Work out the finished part from the listing and answer in its coordinate system (mm). Face numbers are marked on the shaded views. A direction names the side the tool comes from. Give positions to 0.01 mm unless a question says otherwise; leave off trailing zeros. Write each loop counter-clockwise with the first axis right and the second up, starting at its lowest first coordinate (ties: lowest second). Pieces come first, ordered by that corner, then holes.
1) Given pin 1 Ø3 at (y, z) = (6, -1) entering from +X; pin 2 Ø1 at (y, z) = (3.5, 0.5) entering from -X; pin 3 Ø1.5 at (x, z) = (-0.5, -1) entering from +Y, each flat-ended and moving along its own axis, determine where each tip first touches the part or whether it passes through.
2) Determine the mould class of the marked faces 3, 4 and 5 for opening direction Z: pulls with the +Z half, pulls with the -Z half, needs draft (parallel to the pull), parting line crosses it, or undercut.
3) A tool of negligible diameter and unlimited length cuts with its end or side. For the marked faces 1 and 2, from which of +Z, -Z, +X, -X, +Y, -Y can it reach the whole face along a straight path? Write none if from no direction.
4) Find section A-A (y = 14.5). Determine the outline of the cut face in (x, z).
5) Straight lines are drawn through the part: probe 1 along Z at (x, y) = (0, 13); probe 2 along X at (y, z) = (0.25, 3.5); probe 3 along Z at (x, y) = (0, 0). For each, find the intervals that lie inside material, in ascending order.
```python
from build123d import *

# Parameters (mm, degrees)
F9_R          = 2.5
F10_DEPTH     = 15.5
F11_DEPTH     = 4.5
F12_DEPTH     = 6.5
F13_T2_ANGLE  = 157.8095212227
F13_T6_DEPTH  = 3.4652909658
F13_S7_R      = 4.5
F13_T8_DEPTH  = 3
F13_T12_DEPTH = 3.4652909658
F13_S13_R     = 4.5
F13_T14_DEPTH = 3
F13_T16_ANGLE = 157.8095212227
F13_T20_DEPTH = 3.4652909658
F13_S21_R     = 4.5
F13_T22_DEPTH = 3
F13_T26_DEPTH = 3.4652909658
F13_S27_R     = 4.5
F13_T28_DEPTH = 3


# Not quite as in the source:
# - a fillet or chamfer that OpenCascade refuses, or shapes differently, is made with other operations: its cross-section is extruded or revolved along the edge and cut away or added


with BuildPart() as f7:
    # F6 (on Top) → F7 (revolve)
    with BuildSketch(Plane.XY):
        with BuildLine():
            Line((-4, 4.5), (-4, 2.5))
            Line((-4, 2.5), (4, 2.5))
            Line((4, 2.5), (4, 4.5))
            ThreePointArc((4, 4.5), (3.5461149614, 5.1104772433), (3, 5.6400549446))
            ThreePointArc((3, 5.6400549446), (0, 6.716990566), (-3, 5.6400549446))
            ThreePointArc((-3, 5.6400549446), (-3.5461149614, 5.1104772433), (-4, 4.5))
        make_face()
        with BuildLine():
            Line((-3, 7.1961524227), (-3, 5.6400549446))
            ThreePointArc((-3, 5.6400549446), (0, 6.716990566), (3, 5.6400549446))
            Line((3, 5.6400549446), (3, 7.1961524227))
            ThreePointArc((3, 7.1961524227), (0, 8), (-3, 7.1961524227))
        make_face()
    revolve(axis=Axis((0, 0, 0), (1, 0, 0)))

    # F9 (on offset) → F10 (join)
    with BuildSketch(Plane.XZ.offset(-18)):
        with BuildLine():
            ThreePointArc((-4.5, 0), (0, -4.5), (4.5, 0))
            ThreePointArc((4.5, 0), (0, 4.5), (-4.5, 0))
        make_face()
        Circle(F9_R, mode=Mode.SUBTRACT)
        Circle(F9_R)
    extrude(amount=F10_DEPTH)

    # F9 (on offset) → F11 (join)
    with BuildSketch(Plane.XZ.offset(-18)):
        with BuildLine():
            ThreePointArc((-4.5, 0), (0, 4.5), (4.5, 0))
            Line((4.5, 0), (4.5, 2.1794494718))
            ThreePointArc((4.5, 2.1794494718), (0, 5), (-4.5, 2.1794494718))
            Line((-4.5, 2.1794494718), (-4.5, 0))
        make_face()
        with BuildLine():
            Line((4.5, -2.1794494718), (4.5, 0))
            ThreePointArc((4.5, 0), (0, -4.5), (-4.5, 0))
            Line((-4.5, 0), (-4.5, -2.1794494718))
            ThreePointArc((-4.5, -2.1794494718), (0, -5), (4.5, -2.1794494718))
        make_face()
    extrude(amount=F11_DEPTH)

    # F9 (on offset) → F12 (cut)
    with BuildSketch(Plane.XZ.offset(-18)):
        Circle(F9_R)
    extrude(amount=F12_DEPTH, mode=Mode.SUBTRACT)

    # F13: chamfer of 0.5 on 6 edges, made by hand

    # F13_s1 → F13_t2 (revolve, cut)
    with BuildSketch(Plane(origin=(0, 0, 0), x_dir=(0, 1, 0), z_dir=(0.1924404319, 0, -0.9813086569))):
        Polygon((13.5, 4.5), (14, 5), (13.5, 5), align=None)
    revolve(axis=Axis((0, 13.5, 0), (0, -1, 0)), revolution_arc=F13_T2_ANGLE, mode=Mode.SUBTRACT)


with BuildPart() as f13_tool4:
    # F13_s5 → F13_t6 (new body)
    with BuildSketch(Plane.XY):
        Polygon((4, 13.5), (4.5, 14), (4.5, 13.5), align=None)
    extrude(amount=F13_T6_DEPTH)

    # F13_s7 → F13_t8 (cut, symmetric)
    with BuildSketch(Plane.XZ.offset(-13.8)):
        Circle(F13_S7_R)
    extrude(amount=F13_T8_DEPTH, both=True, mode=Mode.SUBTRACT)


with BuildPart() as f7_1:
    add(f7.part)

    # F13_t3: cut F13_tool4
    add(f13_tool4.part, mode=Mode.SUBTRACT)


with BuildPart() as f13_tool10:
    # F13_s11 → F13_t12 (new body)
    with BuildSketch(Plane.XY.offset(3.4652909658)):
        Polygon((-4, 13.5), (-4.5, 14), (-4.5, 13.5), align=None)
    extrude(amount=-F13_T12_DEPTH)

    # F13_s13 → F13_t14 (cut, symmetric)
    with BuildSketch(Plane.XZ.offset(-13.8)):
        Circle(F13_S13_R)
    extrude(amount=F13_T14_DEPTH, both=True, mode=Mode.SUBTRACT)


with BuildPart() as f7_2:
    add(f7_1.part)

    # F13_t9: cut F13_tool10
    add(f13_tool10.part, mode=Mode.SUBTRACT)

    # F13_s15 → F13_t16 (revolve, cut)
    with BuildSketch(Plane(origin=(0, 0, 0), x_dir=(0, 1, 0), z_dir=(-0.1924404319, 0, 0.9813086569))):
        Polygon((13.5, 4.5), (14, 5), (13.5, 5), align=None)
    revolve(axis=Axis((0, 13.5, 0), (0, -1, 0)), revolution_arc=F13_T16_ANGLE, mode=Mode.SUBTRACT)


with BuildPart() as f13_tool18:
    # F13_s19 → F13_t20 (new body)
    with BuildSketch(Plane.XY.offset(-3.4652909658)):
        Polygon((4, 13.5), (4.5, 14), (4.5, 13.5), align=None)
    extrude(amount=F13_T20_DEPTH)

    # F13_s21 → F13_t22 (cut, symmetric)
    with BuildSketch(Plane.XZ.offset(-13.8)):
        Circle(F13_S21_R)
    extrude(amount=F13_T22_DEPTH, both=True, mode=Mode.SUBTRACT)


with BuildPart() as f7_3:
    add(f7_2.part)

    # F13_t17: cut F13_tool18
    add(f13_tool18.part, mode=Mode.SUBTRACT)


with BuildPart() as f13_tool24:
    # F13_s25 → F13_t26 (new body)
    with BuildSketch(Plane.XY):
        Polygon((-4, 13.5), (-4.5, 14), (-4.5, 13.5), align=None)
    extrude(amount=-F13_T26_DEPTH)

    # F13_s27 → F13_t28 (cut, symmetric)
    with BuildSketch(Plane.XZ.offset(-13.8)):
        Circle(F13_S27_R)
    extrude(amount=F13_T28_DEPTH, both=True, mode=Mode.SUBTRACT)


with BuildPart() as f7_4:
    add(f7_3.part)

    # F13_t23: cut F13_tool24
    add(f13_tool24.part, mode=Mode.SUBTRACT)

    # F6 (on Top) → F14 (revolve, cut)
    with BuildSketch(Plane.XY):
        with BuildLine():
            Line((4, 4.5), (4, 2.5))
            Line((4, 2.5), (6, 2.5))
            Line((6, 2.5), (6, 11.5))
            Line((6, 11.5), (4.566472411, 11.5))
            Line((4.566472411, 11.5), (3, 7.1961524227))
            Line((3, 7.1961524227), (3, 5.6400549446))
            ThreePointArc((3, 5.6400549446), (3.5461149614, 5.1104772433), (4, 4.5))
        make_face()
        with BuildLine():
            Line((-6, 2.5), (-4, 2.5))
            Line((-4, 2.5), (-4, 4.5))
            ThreePointArc((-4, 4.5), (-3.5461149614, 5.1104772433), (-3, 5.6400549446))
            Line((-3, 5.6400549446), (-3, 7.1961524227))
            Line((-3, 7.1961524227), (-4.566472411, 11.5))
            Line((-4.566472411, 11.5), (-6, 11.5))
            Line((-6, 11.5), (-6, 2.5))
        make_face()
    revolve(axis=Axis((0, 0, 0), (1, 0, 0)), mode=Mode.SUBTRACT)


solid = f7_4.part
```
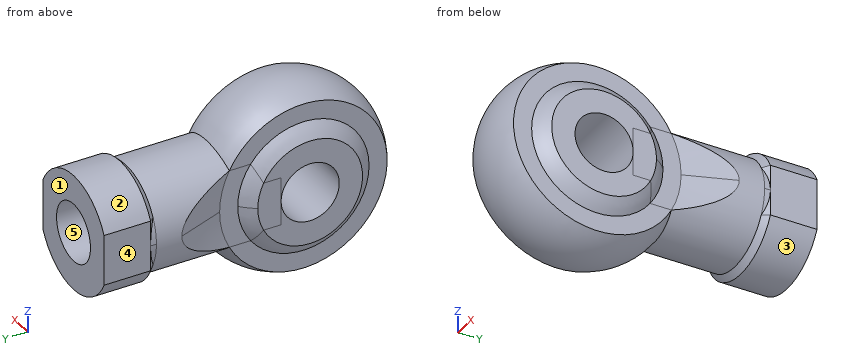
Results:
1. pin 1: stops at x = 3.95
1. pin 2: stops at x = -4
1. pin 3: stops at y = 11.5
2. face 3: pulls with the -Z half
2. face 4: needs draft
2. face 5: undercut
3. face 1: +Z, -Z, +X, -X, +Y
3. face 2: +Z, +Y
4. outline: (-4.5, -2.18) arc R5 ccw to (4.5, -2.18) - (4.5, 2.18) arc R5 ccw to (-4.5, 2.18) - close; hole circle Ø5 at (0, 0)
5. probe 1: z = -4.5 to -2.5, 2.5 to 4.5
5. probe 2: x = -4 to 4
5. probe 3: z = -8 to -2.5, 2.5 to 8
